Can you work these out from the model? Positions are in its coordinate system, mm. A direction names the side the tool comes from. Give positions to 0.01 mm unless a question says otherwise; leave off trailing zeros. Answer as CSV lines item,"result".
```python
from build123d import *

# Parameters (mm, degrees)
F0_W     = 1.15
F0_H     = 3
F0_W_2   = 3
F0_H_2   = 1.15
F1_DEPTH = 160
F2_R     = 5
F4_DEPTH = 200


with BuildPart() as f1:
    # F0 (on Top) → F1 (new body)
    with BuildSketch(Plane.XY):
        with BuildLine():
            Line((7.5, 7.5), (15, 15))
            Line((15, 15), (2.85, 15))
            Line((2.85, 15), (2.85, 12))
            Line((2.85, 12), (2.85, 7))
            Line((2.85, 7), (0, 7))
            Line((0, 7), (0, 1.55))
            ThreePointArc((0, 1.55), (0.5931593202, 1.4320132754), (1.0960155108, 1.0960155108))
            Line((1.0960155108, 1.0960155108), (7.5, 7.5))
        make_face()
        with BuildLine():
            Line((15, 2.85), (15, 15))
            Line((15, 15), (7.5, 7.5))
            Line((7.5, 7.5), (1.0960155108, 1.0960155108))
            ThreePointArc((1.0960155108, 1.0960155108), (1.4320132754, 0.5931593202), (1.55, 0))
            ThreePointArc((1.55, 0), (1.4320132754, -0.5931593202), (1.0960155108, -1.0960155108))
            Line((1.0960155108, -1.0960155108), (7.5, -7.5))
            Line((7.5, -7.5), (15, -15))
            Line((15, -15), (15, -2.85))
            Line((15, -2.85), (12, -2.85))
            Line((12, -2.85), (7, -2.85))
            Line((7, -2.85), (7, 2.85))
            Line((7, 2.85), (12, 2.85))
            Line((12, 2.85), (15, 2.85))
        make_face()
        with Locations((2.275, 13.5)):
            Rectangle(F0_W, F0_H)
        with Locations((13.5, 2.275)):
            Rectangle(F0_W_2, F0_H_2)
        with BuildLine():
            ThreePointArc((-1.0960155108, 1.0960155108), (-0.5931593202, 1.4320132754), (0, 1.55))
            Line((0, 1.55), (0, 7))
            Line((0, 7), (-2.85, 7))
            Line((-2.85, 7), (-2.85, 12))
            Line((-2.85, 12), (-2.85, 15))
            Line((-2.85, 15), (-15, 15))
            Line((-15, 15), (-7.5, 7.5))
            Line((-7.5, 7.5), (-1.0960155108, 1.0960155108))
        make_face()
        with Locations((-2.275, 13.5)):
            Rectangle(F0_W, F0_H)
        with Locations((13.5, -2.275)):
            Rectangle(F0_W_2, F0_H_2)
        with BuildLine():
            Line((7.5, -7.5), (1.0960155108, -1.0960155108))
            ThreePointArc((1.0960155108, -1.0960155108), (0, -1.55), (-1.0960155108, -1.0960155108))
            Line((-1.0960155108, -1.0960155108), (-7.5, -7.5))
            Line((-7.5, -7.5), (-15, -15))
            Line((-15, -15), (-2.85, -15))
            Line((-2.85, -15), (-2.85, -12))
            Line((-2.85, -12), (-2.85, -7))
            Line((-2.85, -7), (2.85, -7))
            Line((2.85, -7), (2.85, -12))
            Line((2.85, -12), (2.85, -15))
            Line((2.85, -15), (15, -15))
            Line((15, -15), (7.5, -7.5))
        make_face()
        with BuildLine():
            ThreePointArc((-1.0960155108, -1.0960155108), (-1.55, 0), (-1.0960155108, 1.0960155108))
            Line((-1.0960155108, 1.0960155108), (-7.5, 7.5))
            Line((-7.5, 7.5), (-15, 15))
            Line((-15, 15), (-15, 2.85))
            Line((-15, 2.85), (-12, 2.85))
            Line((-12, 2.85), (-7, 2.85))
            Line((-7, 2.85), (-7, -2.85))
            Line((-7, -2.85), (-12, -2.85))
            Line((-12, -2.85), (-15, -2.85))
            Line((-15, -2.85), (-15, -15))
            Line((-15, -15), (-7.5, -7.5))
            Line((-7.5, -7.5), (-1.0960155108, -1.0960155108))
        make_face()
        with Locations((-13.5, 2.275)):
            Rectangle(F0_W_2, F0_H_2)
        with Locations((2.275, -13.5)):
            Rectangle(F0_W, F0_H)
        with Locations((-2.275, -13.5)):
            Rectangle(F0_W, F0_H)
        with Locations((-13.5, -2.275)):
            Rectangle(F0_W_2, F0_H_2)
    extrude(amount=F1_DEPTH)

    # F2
    f2_edges = [f1.edges().sort_by_distance(p)[0] for p in [
        (15, -15, 80),
        (-15, -15, 80),
        (15, 15, 80),
        (-15, 15, 80),
    ]]
    fillet(f2_edges, radius=F2_R)

    # F3 (on face) → F4 (cut)
    with BuildSketch(Plane.XY.offset(160)):
        with BuildLine():
            ThreePointArc((-7, -9.5), (-7.1903011687, -8.5432914191), (-7.732233047, -7.732233047))
            Line((-7.732233047, -7.732233047), (-11.267766953, -11.267766953))
            ThreePointArc((-11.267766953, -11.267766953), (-8.5432914191, -11.8096988313), (-7, -9.5))
        make_face()
        with BuildLine():
            Line((-11.267766953, -11.267766953), (-7.732233047, -7.732233047))
            ThreePointArc((-7.732233047, -7.732233047), (-11.267766953, -7.732233047), (-11.267766953, -11.267766953))
        make_face()
        with BuildLine():
            ThreePointArc((11.730266953, -9.230266953), (10.1869755339, -6.9205681217), (7.4625, -7.4625))
            Line((7.4625, -7.4625), (10.9980339059, -10.9980339059))
            ThreePointArc((10.9980339059, -10.9980339059), (11.5399657842, -10.1869755339), (11.730266953, -9.230266953))
        make_face()
        with BuildLine():
            Line((10.9980339059, -10.9980339059), (7.4625, -7.4625))
            ThreePointArc((7.4625, -7.4625), (7.4625, -10.9980339059), (10.9980339059, -10.9980339059))
        make_face()
        with BuildLine():
            ThreePointArc((10.9980339059, 10.9980339059), (7.4625, 10.9980339059), (7.4625, 7.4625))
            Line((7.4625, 7.4625), (10.9980339059, 10.9980339059))
        make_face()
        with BuildLine():
            Line((10.9980339059, 10.9980339059), (7.4625, 7.4625))
            ThreePointArc((7.4625, 7.4625), (10.1869755339, 6.9205681217), (11.730266953, 9.230266953))
            ThreePointArc((11.730266953, 9.230266953), (11.5399657842, 10.1869755339), (10.9980339059, 10.9980339059))
        make_face()
        with BuildLine():
            ThreePointArc((-10.9980339059, 10.9980339059), (-10.9980339059, 7.4625), (-7.4625, 7.4625))
            Line((-7.4625, 7.4625), (-10.9980339059, 10.9980339059))
        make_face()
        with BuildLine():
            Line((-10.9980339059, 10.9980339059), (-7.4625, 7.4625))
            ThreePointArc((-7.4625, 7.4625), (-6.9205681217, 8.2735583721), (-6.730266953, 9.230266953))
            ThreePointArc((-6.730266953, 9.230266953), (-8.2735583721, 11.5399657842), (-10.9980339059, 10.9980339059))
        make_face()
    extrude(amount=-F4_DEPTH, mode=Mode.SUBTRACT)


solid = f1.part
```
Item 1: We'd pull the mould along Y, two halves only. Please class faces 5 (the flat face through (10, -2.85, 79)), 6 (the cylindrical face through (-14, -13, 81)), 7 (the flat face through (0, -3, 160)): released by +Y, released by -Y, zero draft, split by the parting line, or undercut.
Numbers:
face 5,"undercut"
face 6,"released by -Y"
face 7,"zero draft"
Item 2: For faces 1 (the flat face through (-2.85, 9, 79)), 2 (the flat face through (-15, 6, 79)), 3 (the flat face through (-1.7, 13, 79)), 4 (the flat face through (-1.7, -14, 79)), which set-ups out of +Z, -Z, +X, -X, +Y, -Y let a thin tool reach every point of the face, with its end or its side?
Numbers:
face 1,"+Z, -Z"
face 2,"+Z, -Z, -X, +Y, -Y"
face 3,"+Z, -Z, +Y"
face 4,"+Z, -Z, -Y"
Item 3: Please list where these lines run through material, in increasing order: line 1 along Y through (x, z) = (1.75, 29.5); line 2 along Y through (x, z) = (9.5, 47); line 3 along X through (y, z) = (-9.5, 83).
Numbers:
line 1,"y = -15 to -12, -7 to 7, 12 to 15"
line 2,"y = -15 to -11.72, -6.74 to -2.85, 2.85 to 6.74, 11.72 to 15"
line 3,"x = -15 to -12, -7 to -2.85, 2.85 to 6.74, 11.72 to 15"
Item 4: For pin 1 (4 mm diameter, centred on x = 0.5, y = 10, fed in from -Z) (3 decimals); pin 2 (5.5 mm diameter, centred on y = -10.5, z = 85.5, fed in from +X); pin 3 (1.5 mm diameter, centred on x = -14, z = 46, fed in from -Y); pin 4 (3 mm diameter, centred on y = 0, z = 88, fed in from -X), each with a flat end and sliding along its axis, tell me the tip position at first contact or that it passes through.
Numbers:
pin 1,"passes through"
pin 2,"stops at x = 15"
pin 3,"stops at y = -13.8"
pin 4,"stops at x = -7"
Item 5: Imagine slicing it at A-A, the plane z = 115. Give the number of separate pieces and of enclosed holes in the cut face, then the cut area to 3 significant figures.
Numbers:
separate pieces,"1"
enclosed holes,"5"
area,"638 mm²"
